Here's the drawing with two shaded views (mm, measured from the low corner). I have some questions. Round coordinates to 2 decimals unless told otherwise and drop trailing zeros. Loops run counter-clockwise (first coordinate to the right, second up) from the corner with the lowest first, then second, coordinate; pieces in that order, holes last. Notation, with made-up numbers: (76, 18.25) - (121, 18.25) arc R9 ccw to (121, 28.25) - close; hole circle Ø3 at (-23.75, 58.25). An arc over 180 degrees is marked (long way). Use one line per item in the form item = value.
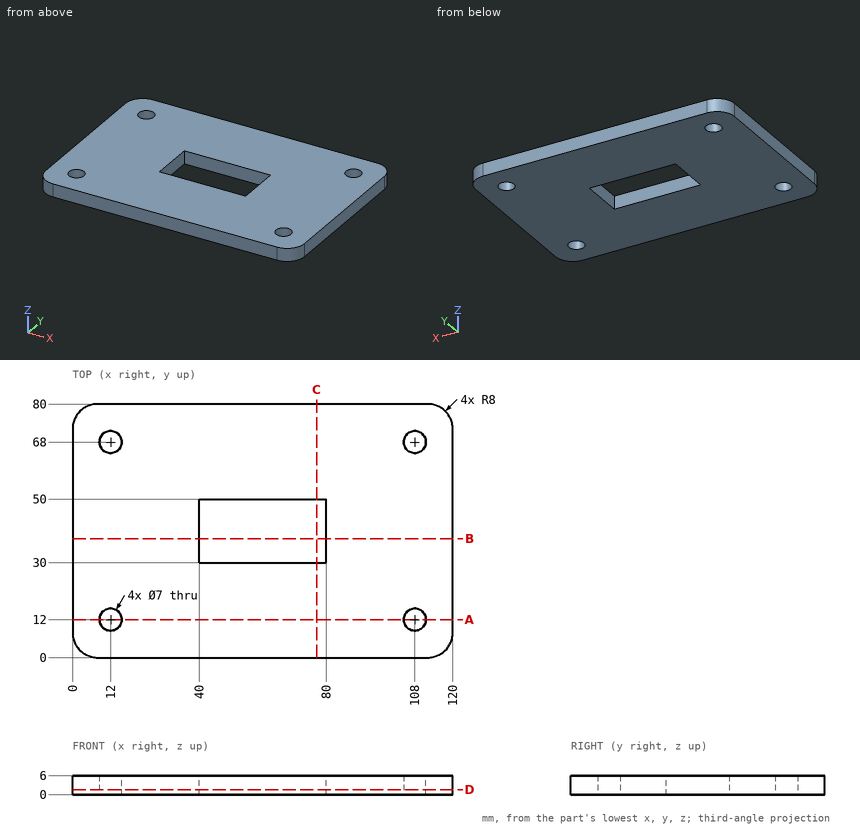
1. If we section it at B-B, the plane y = 37.5: Write out the boundary of the cut face in (x, z).
Solution:
outline = (0, 0) - (40, 0) - (40, 6) - (0, 6) - close; (80, 0) - (120, 0) - (120, 6) - (80, 6) - close
2. If we section it at C-C, the plane x = 77: Write out the boundary of the cut face in (y, z).
Solution:
outline = (0, 0) - (30, 0) - (30, 6) - (0, 6) - close; (50, 0) - (80, 0) - (80, 6) - (50, 6) - close
3. If we section it at D-D, the plane z = 1.55: Write out the boundary of the cut face in (x, y).
Solution:
outline = (0, 8) arc R8 ccw to (8, 0) - (112, 0) arc R8 ccw to (120, 8) - (120, 72) arc R8 ccw to (112, 80) - (8, 80) arc R8 ccw to (0, 72) - close; hole circle Ø7 at (12, 12); hole circle Ø7 at (12, 68); hole (40, 30) - (80, 30) - (80, 50) - (40, 50) - close; hole circle Ø7 at (108, 12); hole circle Ø7 at (108, 68)
4. If we section it at A-A, the plane y = 12: Write out the boundary of the cut face in (x, z).
Solution:
outline = (0, 0) - (8.5, 0) - (8.5, 6) - (0, 6) - close; (15.5, 0) - (104.5, 0) - (104.5, 6) - (15.5, 6) - close; (111.5, 0) - (120, 0) - (120, 6) - (111.5, 6) - close
5. Please list where these lines run through material, in increasing order: line 1 along Y through (x, z) = (12, 4.2); line 2 along X through (y, z) = (12, 2.65); line 3 along X through (y, z) = (48.5, 2.7).
Solution:
line_1 = 0 to 8.5, 15.5 to 64.5, 71.5 to 80
line_2 = 0 to 8.5, 15.5 to 104.5, 111.5 to 120
line_3 = 0 to 40, 80 to 120
